from build123d import *

# Parameters (mm, degrees)
F1_DEPTH = 70


with BuildPart() as f1:
    # F0 (on Front) → F1 (new body)
    with BuildSketch(Plane.XZ):
        with BuildLine():
            Line((0, 34), (0, 12))
            Line((0, 12), (35, 12))
            Line((35, 12), (35, 0))
            Line((35, 0), (80, 0))
            Line((80, 0), (80, 12))
            Line((80, 12), (115, 12))
            Line((115, 12), (115, 34))
            Line((115, 34), (103, 27.071797))
            Line((103, 27.071797), (103, 64.928203))
            Line((103, 64.928203), (115, 58))
            Line((115, 58), (115, 80))
            Line((115, 80), (0, 80))
            Line((0, 80), (0, 58))
            Line((0, 58), (12, 58))
            ThreePointArc((12, 58), (24, 46), (12, 34))
            Line((12, 34), (0, 34))
        make_face()
    extrude(amount=F1_DEPTH)

    # F3 (on face) → F4 section 0
    with BuildSketch(Plane.XZ.offset(70)):
        Polygon((92.5, 80), (22.5, 80), (57.5, 34), align=None)
    # F2 (on face) → F4 section 1
    with BuildSketch(Plane(origin=(0, 0, 0), x_dir=(-1, 0, 0), z_dir=(0, 1, 0))):
        Polygon((-80, 80), (-57.5, 68), (-35, 80), align=None)
    loft(mode=Mode.SUBTRACT)


solid = f1.part
The model under review builds one solid part; all positions refer to its coordinate system, in mm. A direction names the side the tool comes from. Coordinates: 2 decimals unless noted, no trailing zeros. Loops run counter-clockwise (first coordinate to the right, second up) from the corner with the lowest first, then second, coordinate; pieces in that order, holes last.
(1) Consider section A-A, the plane x = 14. Give the boundary of the cut face in (y, z), plus the area to 3 significant figures.
Determined:
outline: (-70, 12) - (0, 12) - (0, 34.17) - (-70, 34.17) - close; (-70, 57.83) - (0, 57.83) - (0, 80) - (-70, 80) - close
area: 3,100 mm2
(2) Consider section B-B, the plane z = 29. Give the boundary of the cut face in (x, y), plus the area to 3 significant figures.
Determined:
outline: (0, -70) - (103, -70) - (103, 0) - (0, 0) - close; (106.34, -70) - (115, -70) - (115, 0) - (106.34, 0) - close
area: 7,820 mm2
(3) Draft analysis for pull direction Z (two halves, no side actions). For faces 1 (the flat face through (6, -35, 34)), 2 (the flat face through (57, 0, 41)), 3 (the flat face through (102, -35, 80)), state which applies: +Z half, -Z half, draft (parallel to the pull), parting line (faces both ways), or undercut.
Determined:
face 1: undercut
face 2: draft
face 3: +Z half
(4) Insertion check: P1, Ø6, axis at x = 7.5, y = -47.5, coming from the -Z side; P2, Ø8, axis at y = -42.5, z = 49.5, coming from the +X side; P3, Ø13, axis at y = -51, z = 5, coming from the -X side. Each pin has a flat end and moves straight along its axis. Give the tip position at first contact, or say it passes through.
Determined:
P1: stops at z = 12
P2: stops at x = 103
P3: stops at x = 35
(5) Wall thickness on L1, parallel to Z at x = 8, y = -24.5; L2, parallel to X at y = -66, z = 62.5; L3, parallel to X at y = -53, z = 33: over which ranges is each line inside the solid? List them lowest first.
Determined:
L1: z = 12 to 34, 58 to 80
L2: x = 0 to 36.83, 78.17 to 103, 107.21 to 115
L3: x = 0 to 103, 113.27 to 115
(6) Tool access review of faces 4 (the flat face through (97, -35, 12)), 5 (the flat face through (35, -35, 6)), 6 (the flat face through (6, -35, 58)): name each direction out of +Z, -Z, +X, -X, +Y, -Y from which nothing blocks a thin tool from reaching the whole face with its end or side.
Determined:
face 4: -Z, +X, +Y, -Y
face 5: -Z, -X, +Y, -Y
face 6: -X, +Y, -Y
